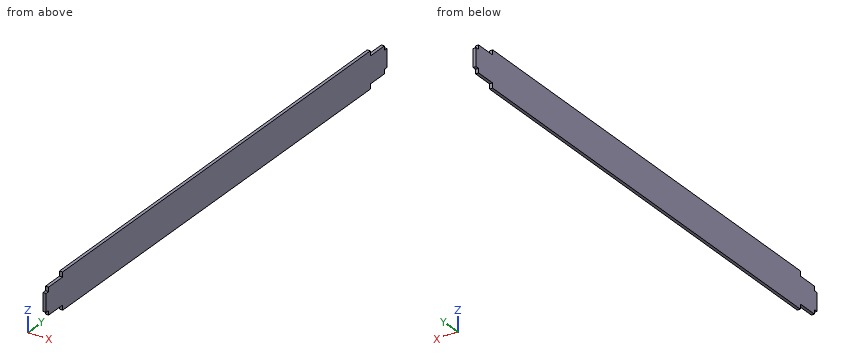
Autodesk Inventor part; units mm, degrees
ref_plane "YZ Plane" through (0, 0, 0) normal (1, 0, 0) x (0, 1, 0)
ref_plane "XZ Plane" through (0, 0, 0) normal (0, 1, 0) x (-1, 0, 0)
ref_plane "XY Plane" through (0, 0, 0) normal (0, 0, 1) x (1, 0, 0)
sketch "Sketch1" plane through (0, 0, 0) normal (1, 0, 0) x (0, 1, 0)
  line L0 (0, 0) -> (822, 0)
  line L1 (822, 0) -> (822, -59.5)
  line L2 (822, -59.5) -> (0, -59.5)
  line L3 (0, -59.5) -> (0, 0)
  line L4 (822, 0) -> (815.75, 0)
  line L5 (815.75, 0) -> (815.75, -15)
  line L6 (815.75, -15) -> (822, -15)
  line L7 (822, -15) -> (822, 0)
  line L8 (822, 0) -> (782, 0)
  line L9 (782, 0) -> (782, -8)
  line L10 (782, -8) -> (822, -8)
  line L11 (822, -8) -> (822, 0)
  line L12 (856.5319, -29.75) -> (-65.1606, -29.75) construction
  line L13 (411, 165.682) -> (411, -1074.2454) construction
  line L14 (822, -59.5) -> (815.75, -59.5)
  line L15 (815.75, -59.5) -> (815.75, -44.5)
  line L16 (815.75, -44.5) -> (822, -44.5)
  line L17 (822, -44.5) -> (822, -59.5)
  line L18 (822, -59.5) -> (782, -59.5)
  line L19 (782, -59.5) -> (782, -51.5)
  line L20 (782, -51.5) -> (822, -51.5)
  line L21 (822, -51.5) -> (822, -59.5)
  line L22 (0, 0) -> (0, -59.5)
  line L23 (0, 0) -> (6.25, 0)
  line L24 (6.25, 0) -> (6.25, -15)
  line L25 (6.25, -15) -> (0, -15)
  line L26 (0, -15) -> (0, 0)
  line L27 (0, 0) -> (40, 0)
  line L28 (40, 0) -> (40, -8)
  line L29 (40, -8) -> (0, -8)
  line L30 (0, -8) -> (0, 0)
  line L31 (6.25, -44.5) -> (0, -44.5)
  line L32 (40, -51.5) -> (0, -51.5)
  line L33 (0, -59.5) -> (6.25, -59.5)
  line L34 (6.25, -59.5) -> (6.25, -44.5)
  line L35 (0, -44.5) -> (0, -59.5)
  line L36 (0, -59.5) -> (40, -59.5)
  line L37 (40, -59.5) -> (40, -51.5)
  line L38 (0, -51.5) -> (0, -59.5)
  point P0 (40, -59.5)
  point P1 (782, -59.5)
  point P2 (815.75, -51.5)
  point P3 (822, -44.5)
  point P4 (822, -15)
  point P5 (815.75, -8)
  point P6 (782, 0)
  point P7 (40, 0)
  point P8 (6.25, -8)
  point P9 (0, -15)
  point P10 (0, -44.5)
  point P11 (6.25, -51.5)
  dimension "d0" = 822
  dimension "d1" = 59.5
  dimension "d2" = 15
  dimension "d3" = 40
  dimension "d4" = 8
  dimension "d5" = 6.25
  dimension "d6" = 29.75
  dimension "d7" = 411
extrude "Extrusion1" add sketch "Sketch1" along normal blind 5 contours L0 L9 L10 L5 L6 L1 L16 L15 L20 L19 L2 L37 L32 L34 L31 L3 L25 L24 L29 L28
equation "\"d6\" = 0.5 * d1"
equation "\"d7\" = 0.5 * d0"
properties part number "Acrly_Wand_1"
Geometry: final body of the model. Coordinates: model frame, mm. Give positions to 0.01 mm unless a question says otherwise; leave off trailing zeros. Order: outer loops, then holes, each group sorted by start corner. A loop starts at its lowest first (then second) coordinate and runs counter-clockwise, first axis right, second up. Notation, with made-up numbers: (21, 75) -> (63, 75) arc R14 cw to (63, 82) -> close; hole circle Ø2 at (5, 25.5). An arc over 180 degrees is marked (long way). Answer as a JSON object with one key per item and string values.
Q1. First-contact query: pin 1 (2.5 mm diameter, centred on x = 2, z = -6, fed in from +Y); pin 2 (1.5 mm diameter, centred on x = 2.5, z = -13, fed in from -Y); pin 3 (2.5 mm diameter, centred on x = 2.5, z = -57, fed in from -Y). Flat tips, straight axial feed; report the tip coordinate or a pass-through.
Entries:
{"pin 1": "stops at y = 782", "pin 2": "stops at y = 6.25", "pin 3": "stops at y = 40"}
Q2. Material intervals for probe 1 along Y at (x, z) = (0.5, -13); probe 2 along Y at (x, z) = (1.4, -55.5), sorted ascending.
Entries:
{"probe 1": "y = 6.25 to 815.75", "probe 2": "y = 40 to 782"}
Q3. Section A-A (x = 1.8). Output: boundary loops of the cut face in (y, z), plus the area to 3 significant figures.
Entries:
{"outline": "(0, -44.5) -> (6.25, -44.5) -> (6.25, -51.5) -> (40, -51.5) -> (40, -59.5) -> (782, -59.5) -> (782, -51.5) -> (815.75, -51.5) -> (815.75, -44.5) -> (822, -44.5) -> (822, -15) -> (815.75, -15) -> (815.75, -8) -> (782, -8) -> (782, 0) -> (40, 0) -> (40, -8) -> (6.25, -8) -> (6.25, -15) -> (0, -15) -> close", "area": "47,500 mm^2"}
